```python
from build123d import *

# Parameters (mm, degrees)
SKETCH_1_W          = 40
SKETCH_1_H          = 30
EXTRUDE_1_DEPTH     = 24
SKETCH_2_R          = 1.6
CUT_EXTRUDE_1_DEPTH = 24
SKETCH_3_R          = 2.1
CUT_EXTRUDE_2_DEPTH = 34


with BuildPart() as part:
    # 草图1 → 凸台-拉伸1 (new body)
    with BuildSketch(Plane.XY):
        with Locations((20, -15)):
            Rectangle(SKETCH_1_W, SKETCH_1_H)
    extrude(amount=EXTRUDE_1_DEPTH)

    # 草图2 → 切除-拉伸1 (cut)
    with BuildSketch(Plane(origin=(0, 0, 0), x_dir=(-1, 0, 0), z_dir=(0, 0, -1))):
        with BuildLine():
            ThreePointArc((-14, -20.979949748), (-20, -9.8), (-26, -20.979949748))
            Line((-26, -20.979949748), (-26, -30))
            Line((-26, -30), (-20, -30))
            Line((-20, -30), (-14, -30))
            Line((-14, -30), (-14, -20.979949748))
        make_face()
        with Locations((-10.90673326, -11.75)):
            Circle(SKETCH_2_R)
        with Locations((-10.90673326, -22.25)):
            Circle(SKETCH_2_R)
        with Locations((-29.09326674, -22.25)):
            Circle(SKETCH_2_R)
        with Locations((-29.09326674, -11.75)):
            Circle(SKETCH_2_R)
    extrude(amount=-CUT_EXTRUDE_1_DEPTH, mode=Mode.SUBTRACT)

    # 草图3 → 切除-拉伸2 (cut)
    with BuildSketch(Plane(origin=(0, 0, 0), x_dir=(1, 0, 0), z_dir=(0, 1, 0))):
        with Locations(Location((5, -6, 0), (0, 0, 270))):
            Circle(SKETCH_3_R)
        with Locations(Location((35, -6, 0), (0, 0, 270))):
            Circle(SKETCH_3_R)
        with Locations(Location((5, -18, 0), (0, 0, 270))):
            Circle(SKETCH_3_R)
        with Locations(Location((35, -18, 0), (0, 0, 270))):
            Circle(SKETCH_3_R)
    extrude(amount=-CUT_EXTRUDE_2_DEPTH, mode=Mode.SUBTRACT)


solid = part.part
```
Here's how the part is built. I have some questions about the finished solid (model axes, mm). A direction names the side the tool comes from. Coordinates: 2 decimals unless noted, no trailing zeros. Loops run counter-clockwise (first coordinate to the right, second up) from the corner with the lowest first, then second, coordinate; pieces in that order, holes last. Notation, with made-up numbers: M -26.75,-27 L 0.25,-27 A11 cw 0.25,-15 Z; hole C 85,46.5 d11. An arc over 180 degrees is marked long. One line per item, written item: value.
1. Imagine slicing it at B-B (z = 18). List the corners of the cut face in (x, y) for me, and give its area (3 significant figures).
Geometry says:
outline: M 0,-30 L 2.9,-30 L 2.9,0 L 0,0 Z; M 7.1,-30 L 14,-30 L 14,-20.98 A7.2 cw long 26,-20.98 L 26,-30 L 32.9,-30 L 32.9,0 L 7.1,0 Z; M 37.1,-30 L 40,-30 L 40,0 L 37.1,0 Z; hole C 10.91,-22.25 d3.2; hole C 10.91,-11.75 d3.2; hole C 29.09,-22.25 d3.2; hole C 29.09,-11.75 d3.2
area: 672 mm2
2. Will this pin go through, and if not, where does the flat tip stop? pin 1 Ø3 at (x, y) = (29.09, -22.25) entering from -Z.
Geometry says:
pin 1: passes through
3. Please list where these lines run through material, in increasing order: probe 1 along X at (y, z) = (-26.75, 6); probe 2 along X at (y, z) = (-6.5, 18); probe 3 along Y at (x, z) = (11, 14.5).
Geometry says:
probe 1: x = 0 to 2.9, 7.1 to 14, 26 to 32.9, 37.1 to 40
probe 2: x = 0 to 2.9, 7.1 to 32.9, 37.1 to 40
probe 3: y = -30 to -23.85, -20.65 to -13.35, -10.15 to 0
4. Thinking about a two-plate mould opening in X: for faces 1 (the flat face through (15, -11, 24)), 2 (the flat face through (40, -15, 12)), 3 (the flat face through (26, -25, 12)), which applies, +X half, -X half, draft (parallel to the pull), parting line (faces both ways), or undercut?
Geometry says:
face 1: draft
face 2: +X half
face 3: undercut
5. Imagine slicing it at D-D (y = -17). List the corners of the cut face in (x, z) for me, and give its area (3 significant figures).
Geometry says:
outline: M 0,0 L 12.8,0 L 12.8,24 L 0,24 Z; M 27.2,0 L 40,0 L 40,24 L 27.2,24 Z; hole C 5,6 d4.2; hole C 5,18 d4.2; hole C 35,6 d4.2; hole C 35,18 d4.2
area: 559 mm2
6. Imagine slicing it at C-C (x = 35). List the corners of the cut face in (y, z) for me, and give its area (3 significant figures).
Geometry says:
outline: M -30,0 L 0,0 L 0,3.9 L -30,3.9 Z; M -30,8.1 L 0,8.1 L 0,15.9 L -30,15.9 Z; M -30,20.1 L 0,20.1 L 0,24 L -30,24 Z
area: 468 mm2
7. On a 3-axis mill with a long thin cutter (end or side, diameter ignored), from which of +Z, -Z, +X, -X, +Y, -Y can I reach the whole of each face in a straight line? I mean faces 4 (the flat face through (14, -26, 12)), 5 (the flat face through (0, -15, 12)). Say none if no direction works.
Geometry says:
face 4: +Z, -Z, -Y
face 5: +Z, -Z, -X, +Y, -Y
8. Imagine slicing it at A-A (y = -22.25). List the corners of the cut face in (x, z) for me, and give its area (3 significant figures).
Geometry says:
outline: M 0,0 L 9.31,0 L 9.31,24 L 0,24 Z; M 12.51,0 L 14,0 L 14,24 L 12.51,24 Z; M 26,0 L 27.49,0 L 27.49,24 L 26,24 Z; M 30.69,0 L 40,0 L 40,24 L 30.69,24 Z; hole C 5,6 d4.2; hole C 5,18 d4.2; hole C 35,6 d4.2; hole C 35,18 d4.2
area: 463 mm2
